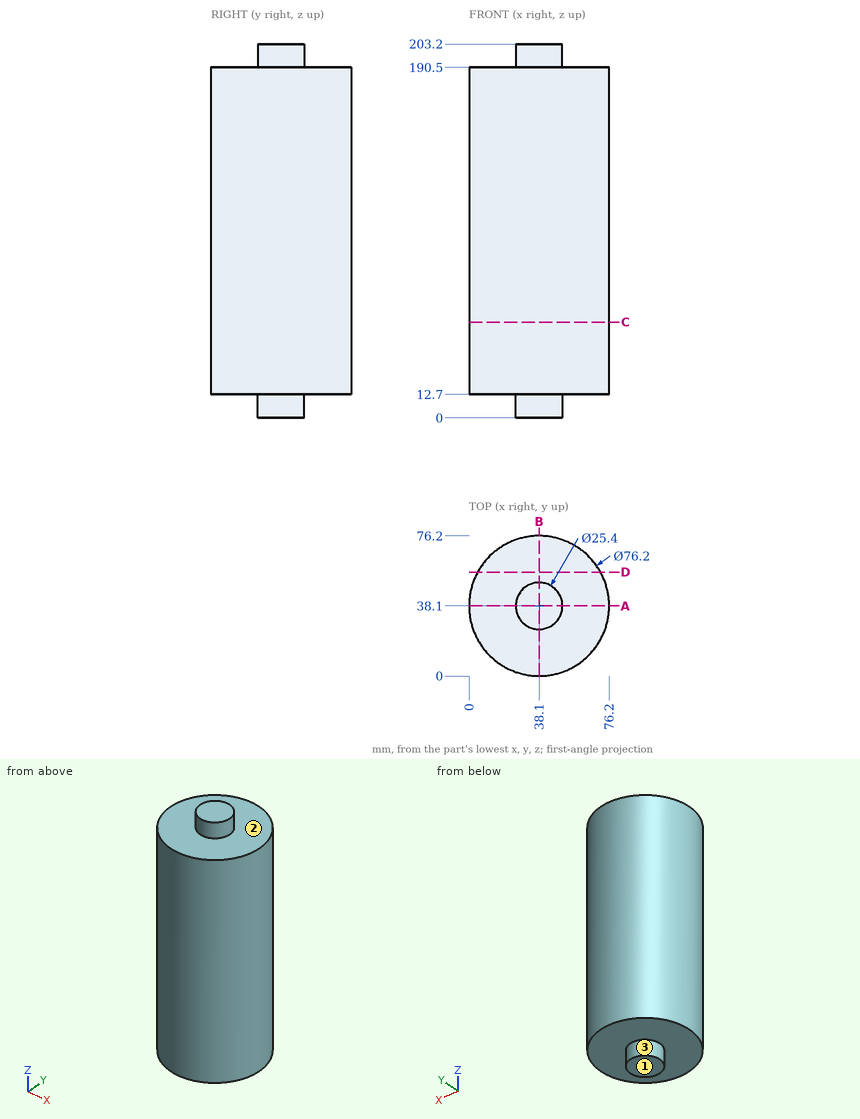
Input: dimensioned drawing with shaded views. Units: mm. Origin: part minimum x, y, z. A direction names the side the tool comes from. Coordinates: 2 decimals unless noted, no trailing zeros. Loops run counter-clockwise (first coordinate to the right, second up) from the corner with the lowest first, then second, coordinate; pieces in that order, holes last. Notation, with made-up numbers: M 56.5,-3.75 L 62.5,-3.75 A19 ccw 62.5,11.25 Z; hole C 40.5,-29 d6. An arc over 180 degrees is marked long. Use a Markdown table: item, result. Add a question column.
1) Line query: L1, parallel to Z at x = 63.5, y = 25; L2, parallel to Y at x = 68.5, z = 106.5; L3, parallel to Y at x = 44.5, z = 70. Output: solid intervals per line, ascending. Write a range as from..to.
2) Section D-D, the plane y = 56.5. Return the cut outline in (x, z), plus the area to 3 significant figures.
3) Section C-C, the plane z = 52. Return the cut outline in (x, y), plus the area to 3 significant figures.
4) Section A-A, the plane y = 38.1. Return the cut outline in (x, z), plus the area to 3 significant figures.
5) Set-up query: the marked faces 1, 2 and 3. Return all of +Z, -Z, +X, -X, +Y, -Y with unobstructed straight access to the full face (end or side cutting, diameter ignored); none if empty.
6) Pin query (flat end, axial travel): P1, Ø2, axis at y = 53, z = 126, coming from the +X side; P2, Ø3, axis at x = 67.5, y = 56.5, coming from the +Z side; P3, Ø1.5, axis at y = 60.5, z = 51, coming from the +X side. Return the tip coordinate at first contact, or that it passes through.
Answer below:
| question | item | result |
|---|---|---|
| 1 | L1 | 12.7..190.5 |
| 1 | L2 | 15.13..61.07 |
| 1 | L3 | 0.54..75.66 |
| 2 | outline | M 4.74,12.7 L 71.46,12.7 L 71.46,190.5 L 4.74,190.5 Z |
| 2 | area | 11,900 mm2 |
| 3 | outline | C 38.1,38.1 d76.2 |
| 3 | area | 4,560 mm2 |
| 4 | outline | M 0,12.7 L 25.4,12.7 L 25.4,0 L 50.8,0 L 50.8,12.7 L 76.2,12.7 L 76.2,190.5 L 50.8,190.5 L 50.8,203.2 L 25.4,203.2 L 25.4,190.5 L 0,190.5 Z |
| 4 | area | 14,200 mm2 |
| 5 | face 1 | -Z, +X, -X, +Y, -Y |
| 5 | face 2 | +Z |
| 5 | face 3 | -Z |
| 6 | P1 | x = 73.57 |
| 6 | P2 | z = 190.5 |
| 6 | P3 | x = 69.45 |
